Build history of the part. All positions in model axes, mm. Round coordinates to 2 decimals unless told otherwise and drop trailing zeros. Loops run counter-clockwise (first coordinate to the right, second up) from the corner with the lowest first, then second, coordinate; pieces in that order, holes last.
from build123d import *

# Parameters (mm, degrees)
F1_DEPTH = 100
F2_W     = 3.295
F2_H     = 4.472
F3_DEPTH = 80
F4_W     = 3.295
F4_H     = 4.472
F5_DEPTH = 80
F7_DEPTH = 25
F9_DEPTH = 25


with BuildPart() as f1:
    # F0 (on Top) → F1 (new body)
    with BuildSketch(Plane.XY):
        Polygon((103.941999, 2.236), (-26.058001, 2.236), (-26.058001, 0), (-26.058001, -2.236), (103.941999, -2.236), (103.941999, 0), align=None)
    extrude(amount=F1_DEPTH)

    # F2 (on face) → F3 (cut)
    with BuildSketch(Plane(origin=(0, 0, 0), x_dir=(1, 0, 0), z_dir=(0, 0, -1))):
        with Locations((-21.057501, 0)):
            Rectangle(F2_W, F2_H)
    extrude(amount=-F3_DEPTH, mode=Mode.SUBTRACT)

    # F4 (on face) → F5 (cut)
    with BuildSketch(Plane(origin=(0, 0, 0), x_dir=(1, 0, 0), z_dir=(0, 0, -1))):
        with Locations((98.941499, 0)):
            Rectangle(F4_W, F4_H)
    extrude(amount=-F5_DEPTH, mode=Mode.SUBTRACT)

    # F6 (on face) → F7 (cut)
    with BuildSketch(Plane.XZ.offset(2.236)):
        Polygon((-22.705001, 3.723884), (-26.058001, 0), (-22.705001, 0), align=None)
        Polygon((-16.057001, 0), (-19.410001, 3.723884), (-19.410001, 0), align=None)
    extrude(amount=-F7_DEPTH, mode=Mode.SUBTRACT)

    # F8 (on face) → F9 (cut)
    with BuildSketch(Plane.XZ.offset(2.236)):
        Polygon((97.293999, 0), (97.293999, 3.723884), (93.940999, 0), align=None)
        Polygon((100.588999, 0), (103.941999, 0), (100.588999, 3.723884), align=None)
    extrude(amount=-F9_DEPTH, mode=Mode.SUBTRACT)


solid = f1.part
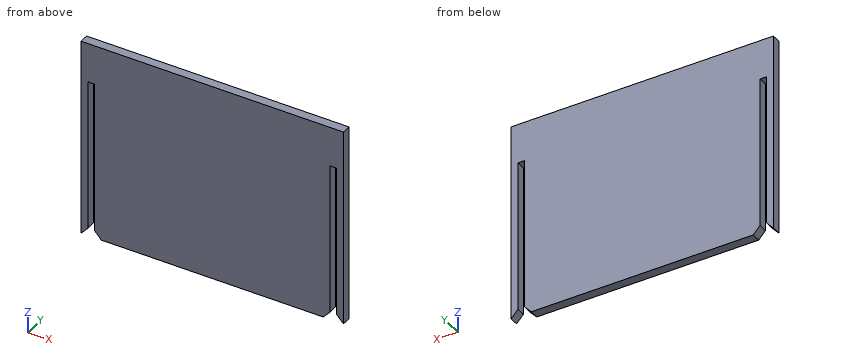
(1) Slice it at A-A on z = 63. List the corners of the cut face in (x, y) (3 decimals), plus the area to 3 significant figures.
Responses:
outline: (-26.058, -2.236) - (-22.705, -2.236) - (-22.705, 2.236) - (-26.058, 2.236) - close; (-19.41, -2.236) - (97.294, -2.236) - (97.294, 2.236) - (-19.41, 2.236) - close; (100.589, -2.236) - (103.942, -2.236) - (103.942, 2.236) - (100.589, 2.236) - close
area: 552 mm2
(2) Probe line 1 (X direction, y = 1.8, z = 60.5) (3 decimals); line 2 (Z direction, x = 98, y = 1.6); line 3 (Z direction, x = 96, y = 0.3). List the from-to ranges inside material, lowest first.
Responses:
line 1: x = -26.058 to -22.705, -19.41 to 97.294, 100.589 to 103.942
line 2: z = 80 to 100
line 3: z = 2.29 to 100
(3) Slice it at B-B on y = -0.4. List the corners of the cut face in (x, z) (3 decimals), plus the area to 3 significant figures.
Responses:
outline: (-26.058, 0) - (-22.705, 3.724) - (-22.705, 80) - (-19.41, 80) - (-19.41, 3.724) - (-16.057, 0) - (93.941, 0) - (97.294, 3.724) - (97.294, 80) - (100.589, 80) - (100.589, 3.724) - (103.942, 0) - (103.942, 100) - (-26.058, 100) - close
area: 12,400 mm2
(4) Pin check, flat tips, straight feed: P1, Ø2.5, axis at x = 99.5, y = -0.5, coming from the -Z side; P2, Ø1, axis at x = -21.5, y = -0.5, coming from the -Z side. Stop position of each tip, or through.
Responses:
P1: stops at z = 3.55
P2: stops at z = 80
